Model file for the job. Use its own axes, mm. A direction names the side the tool comes from. Give positions to 0.01 mm unless a question says otherwise; leave off trailing zeros. Loops run counter-clockwise (first coordinate to the right, second up) from the corner with the lowest first, then second, coordinate; pieces in that order, holes last. Notation, with made-up numbers: M -10.75,48 L 48.25,48 A8 cw 48.25,60 Z; hole C 81,34 d6. An arc over 180 degrees is marked long. Answer in a Markdown table with one row per item.
```python
from build123d import *

# Parameters (mm, degrees)
F0_R     = 50.8
F1_DEPTH = 6.35
F3_DEPTH = 3.175


with BuildPart() as f1:
    # F0 (on Top) → F1 (new body)
    with BuildSketch(Plane.XY):
        Circle(F0_R)
    extrude(amount=F1_DEPTH)

    # F2 (on face) → F3 (cut)
    with BuildSketch(Plane.XY.offset(6.35)):
        with BuildLine():
            ThreePointArc((7.240724, 38.556855), (-13.52335, 17.681434), (-23.170317, -10.137014))
            ThreePointArc((-23.170317, -10.137014), (1.51189, -38.287895), (24.437444, -8.688869))
            ThreePointArc((24.437444, -8.688869), (20.26616, 2.14385), (13.033303, 11.223122))
            ThreePointArc((13.033303, 11.223122), (6.51881, 24.123217), (7.240724, 38.556855))
        make_face()
        with BuildLine():
            ThreePointArc((14.23507, 0.897387), (18.697847, -4.377114), (20.330649, -11.090585))
            ThreePointArc((20.330649, -11.090585), (19.118678, -15.698466), (14.94622, -17.998908))
            ThreePointArc((14.94622, -17.998908), (11.829196, -16.1818), (11.288874, -12.614479))
            ThreePointArc((11.288874, -12.614479), (14.072181, -6.144231), (14.23507, 0.897387))
        make_face(mode=Mode.SUBTRACT)
    extrude(amount=-F3_DEPTH, mode=Mode.SUBTRACT)


solid = f1.part
```
Q1. Mould opens along Y. For faces 1 (the face through (0.9, -38.3, 4.8)), 2 (the face through (-11.012, -49.592, 3.131)), 3 (the face through (16, -11, 6.35)) say: released by +Y, released by -Y, zero draft, split by the parting line, or undercut.
Reported:
| item | result |
|---|---|
| face 1 | undercut |
| face 2 | split by the parting line |
| face 3 | zero draft |
Q2. 3-axis set-ups, long thin cutter, end or side, ignore diameter. For faces 4 (the face through (19.161, -15.644, 4.785)), 5 (the face through (-1, 1, 0)): which of +Z, -Z, +X, -X, +Y, -Y reach the whole face in a straight line?
Reported:
| item | result |
|---|---|
| face 4 | +Z |
| face 5 | -Z, +X, -X, +Y, -Y |
Q3. Saw through at A-A (y = 20). Give the cut face in (x, z) (3 decimals).
Reported:
| item | result |
|---|---|
| outline | M -46.697,0 L 46.697,0 L 46.697,6.35 L 7.727,6.35 L 7.727,3.175 L -12.007,3.175 L -12.007,6.35 L -46.697,6.35 Z |
Q4. Saw through at B-B (x = 22). Give the cut face in (y, z) (3 decimals), and give its area (3 significant figures).
Reported:
| item | result |
|---|---|
| outline | M -45.789,0 L 45.789,0 L 45.789,6.35 L -1.27,6.35 L -1.27,3.175 L -25.788,3.175 L -25.788,6.35 L -45.789,6.35 Z |
| area | 504 mm² |
Q5. Saw through at D-D (x = 33). Give the cut face in (y, z), and give its area (3 significant figures).
Reported:
| item | result |
|---|---|
| outline | M -38.62,0 L 38.62,0 L 38.62,6.35 L -38.62,6.35 Z |
| area | 490 mm² |
Q6. Drop flat-ended pins along their axis: pin 1 (2 mm diameter, centred on y = -4.5, z = 1.5, fed in from +X); pin 2 (2 mm diameter, centred on x = 2.5, y = 20.5, fed in from +Z) (3 decimals). Give the stop position or say it passes through.
Reported:
| item | result |
|---|---|
| pin 1 | x = 50.68 |
| pin 2 | z = 3.175 |
Q7. Saw through at C-C (z = 1). Give the cut face in (x, y), and give its area (3 significant figures).
Reported:
| item | result |
|---|---|
| outline | C 0,0 d101.6 |
| area | 8,110 mm² |
Q8. Probe probe 1 along X at (y, z) = (-14.5, 3.75); probe 2 along Z at (x, y) = (-9.5, -2) (3 decimals); probe 3 along X at (y, z) = (4, 4.75). List the from-to ranges inside material, lowest first.
Reported:
| item | result |
|---|---|
| probe 1 | -48.69 to -23.48, 11.16 to 19.85, 25.03 to 48.69 |
| probe 2 | 0 to 3.175 |
| probe 3 | -50.64 to -20.02, 19.13 to 50.64 |
